Read the model definition and answer for the solid it produces. Units are mm, in the model's axes. A direction names the side the tool comes from. Coordinates: 2 decimals unless noted, no trailing zeros. Write each loop counter-clockwise with the first axis right and the second up, starting at its lowest first coordinate (ties: lowest second). Pieces come first, ordered by that corner, then holes. Notation, with made-up numbers: (58.25, 45) -> (71.25, 45) arc R32 ccw to (71.25, 80) -> close; hole circle Ø4 at (28.25, 20.5). An arc over 180 degrees is marked (long way). Answer in a Markdown table with one row per item. Add a question column.
Item 1: Straight lines are drawn through the part: line 1 (X direction, y = 1, z = -38); line 2 (X direction, y = 1.5, z = -29); line 3 (Z direction, x = 15, y = 1.5). For each, find the intervals that lie inside material, in ascending order. Write a range as from..to.
Item 2: Section A-A on z = -45 is taken. Write down the section's boundary in (x, y), then the cut area to 3 significant figures.
Item 3: Section B-B on x = 13.5 is taken. Write down the section's boundary in (y, z).
Item 4: Which of the six approach directions +Z, -Z, +X, -X, +Y, -Y give full straight-line access (tool end or side, diameter ignored) to faces 1 (the face through (13, 0, -52)), 2 (the face through (12.5, 1, -18))?
Item 5: Given pin 1 Ø0.5 at (x, y) = (14.5, 0.5) entering from +Z; pin 2 Ø0.9 at (y, z) = (1, -43) entering from +X, each flat-ended and moving along its own axis, determine where each tip first touches the part or whether it passes through.
Item 6: For a pull along Z with two mould halves and no side action, classify faces 3 (the face through (13, 1, -83.5)), 4 (the face through (12, 1, -43)), 5 (the face through (13, 1.8, -52)) as +Z half, -Z half, draft (parallel to the pull), parting line (faces both ways), or undercut.
```python
from build123d import *

# Parameters (mm, degrees)
BOSS_EXTRUDE1_DEPTH = 1.8
FILLET2_R           = 0.5
SKETCH3_R           = 2.5
SKETCH3_R_2         = 1.75
BOSS_EXTRUDE2_DEPTH = 1.8
FILLET3_R           = 1
CUT_EXTRUDE1_DEPTH  = 2.8000001
FILLET4_R           = 0.5


with BuildPart() as part:
    # Sketch1 → Boss-Extrude1 (new body)
    with BuildSketch(Plane(origin=(0, 0, 0), x_dir=(1, 0, 0), z_dir=(0, 1, 0))):
        with BuildLine():
            Line((0, 4.5), (0, 6.5))
            Line((0, 6.5), (6.1, 6.5))
            Line((6.1, 6.5), (6.1, 10.5))
            Line((6.1, 10.5), (10, 14.4))
            Line((10, 14.4), (10, 83.5))
            Line((10, 83.5), (16.4, 83.5))
            ThreePointArc((16.4, 83.5), (17.2719581, 81.425344658), (17.601960582, 79.199226044))
            Line((17.601960582, 79.199226044), (18.25, 49.5))
            Line((18.25, 49.5), (12, 49.5))
            Line((12, 49.5), (12, 37.18))
            add(Edge.make_bspline(
                [(12.5, 32.33), (12.5, 33.972282338), (12, 35.554764974), (12, 37.18)],
                knots=[0, 0, 0, 0, 1, 1, 1, 1], degree=3))
            Line((12.5, 32.33), (12.5, 3.07))
            ThreePointArc((12.5, 3.07), (11.600817818, 0.899182182), (9.43, 0))
            ThreePointArc((9.43, 0), (4.205660329, 1.182650422), (0, 4.5))
        make_face()
    extrude(amount=BOSS_EXTRUDE1_DEPTH)

    # Fillet2
    fillet2_edges = [part.edges().sort_by_distance(p)[0] for p in [
        (0, 0.9, -6.5),
        (6.1, 0.9, -6.5),
        (6.1, 0.9, -10.5),
        (10, 0.9, -14.4),
        (10, 0.9, -83.5),
        (18.25, 0.9, -49.5),
        (12, 0.9, -49.5),
    ]]
    fillet(fillet2_edges, radius=FILLET2_R)

    # Sketch3 → Boss-Extrude2 (add)
    with BuildSketch(Plane.XZ):
        with Locations((9.5, 2.499832541)):
            Circle(SKETCH3_R)
        with Locations((9.5, 2.499832541)):
            Circle(SKETCH3_R_2, mode=Mode.SUBTRACT)
        with BuildLine():
            ThreePointArc((11.824045318, 1.578521867), (9.031018815, 0.044215175), (7, 2.499832541))
            Line((7, 2.499832541), (7, -0.245881701))
            ThreePointArc((7, -0.245881701), (8.2087959, -0.061626967), (9.43, 0))
            ThreePointArc((9.43, 0), (10.256451345, -0.113333266), (11.021883517, -0.444965358))
            Line((11.021883517, -0.444965358), (11.824045318, 1.578521867))
        make_face()
        with BuildLine():
            ThreePointArc((9.43, 0), (8.2087959, -0.061626967), (7, -0.245881701))
            Line((7, -0.245881701), (7, -0.500167459))
            Line((7, -0.500167459), (11, -0.500167459))
            Line((11, -0.500167459), (11.021883517, -0.444965358))
            ThreePointArc((11.021883517, -0.444965358), (10.256451345, -0.113333266), (9.43, 0))
        make_face()
    extrude(amount=-BOSS_EXTRUDE2_DEPTH)

    # Fillet3
    fillet3_edges = [part.edges().sort_by_distance(p)[0] for p in [
        (7, 0.9, -0.245881701),
        (11.021883517, 0.9, -0.444965358),
    ]]
    fillet(fillet3_edges, radius=FILLET3_R)

    # Sketch4 → Cut-Extrude1 (cut, through all)
    with BuildSketch(Plane(origin=(0, 1.8, 0), x_dir=(1, 0, 0), z_dir=(0, 1, 0))):
        Polygon((10, 18.881660772), (10, 3.27), (13.61834734, 3.27), (13.61834734, -6.687183429), (-3.427548793, -6.687183429), (-3.427548793, 18.881660772), align=None)
    extrude(amount=-CUT_EXTRUDE1_DEPTH, mode=Mode.SUBTRACT)

    # Fillet4
    fillet4_edges = [part.edges().sort_by_distance(p)[0] for p in [
        (12.5, 0.9, -3.27),
        (10, 0.9, -3.27),
    ]]
    fillet(fillet4_edges, radius=FILLET4_R)


solid = part.part
```
Results below:
| question | item | result |
|---|---|---|
| 1 | line 1 | x = 10..12 |
| 1 | line 2 | x = 10..12.5 |
| 1 | line 3 | z = -83.5..-49.5 |
| 2 | outline | (10, 0) -> (12, 0) -> (12, 1.8) -> (10, 1.8) -> close |
| 2 | area | 3.60 mm2 |
| 3 | outline | (0, -83.5) -> (1.8, -83.5) -> (1.8, -49.5) -> (0, -49.5) -> close |
| 4 | face 1 | +Z, -Z, +X, -X, -Y |
| 4 | face 2 | +Z, +X, +Y, -Y |
| 5 | pin 1 | stops at z = -49.5 |
| 5 | pin 2 | stops at x = 12 |
| 6 | face 3 | -Z half |
| 6 | face 4 | undercut |
| 6 | face 5 | draft |
